Can you work these out from the model? Positions are in its coordinate system, mm. A direction names the side the tool comes from. Give positions to 0.01 mm unless a question says otherwise; leave off trailing zeros. Loops run counter-clockwise (first coordinate to the right, second up) from the corner with the lowest first, then second, coordinate; pieces in that order, holes last. Notation, with made-up numbers: (51.25, 39) - (107.25, 39) arc R18 cw to (107.25, 48) - close; hole circle Ø5 at (-9, 65.25). An arc over 180 degrees is marked (long way). Answer in a Markdown table with one row per item.
from build123d import *

# Parameters (mm, degrees)
SKETCH4_W                                       = 300
SKETCH4_H                                       = 100
BOSS_EXTRUDE2_DEPTH                             = 20
CSK_FOR_M2_FLAT_HEAD_MACHINE_SCREW1_D           = 2.4
CSK_FOR_M2_FLAT_HEAD_MACHINE_SCREW1_CSINK_D     = 4.4
CSK_FOR_M2_FLAT_HEAD_MACHINE_SCREW1_CSINK_ANGLE = 90
CBORE_FOR_M5_HEX_HEAD_BOLT1_D                   = 5.5
CBORE_FOR_M5_HEX_HEAD_BOLT1_CBORE_D             = 12.24
CBORE_FOR_M5_HEX_HEAD_BOLT1_CBORE_DEPTH         = 3.58


with BuildPart() as part:
    # Sketch4 → Boss-Extrude2 (new body)
    with BuildSketch(Plane(origin=(0, 0, 0), x_dir=(1, 0, 0), z_dir=(0, 1, 0))):
        Rectangle(SKETCH4_W, SKETCH4_H)
    extrude(amount=BOSS_EXTRUDE2_DEPTH)

    # CSK for M2 Flat Head Machine Screw1 (through all)
    with Locations(Plane(origin=(0, 20, 0), x_dir=(1, 0, 0), z_dir=(0, 1, 0))):
        with Locations((-120, 0), (-106, -0.273765591), (-112.818119913, 7.041508898), (-112.818119913, -6.958491102)):
            CounterSinkHole(CSK_FOR_M2_FLAT_HEAD_MACHINE_SCREW1_D / 2, CSK_FOR_M2_FLAT_HEAD_MACHINE_SCREW1_CSINK_D / 2, counter_sink_angle=CSK_FOR_M2_FLAT_HEAD_MACHINE_SCREW1_CSINK_ANGLE)

    # CBORE for M5 Hex Head Bolt1 (through all)
    with Locations(Plane(origin=(0, 0, -50), x_dir=(-1, 0, 0), z_dir=(0, 0, -1))):
        with Locations((0, 10), (-100, 10), (100, 10)):
            CounterBoreHole(CBORE_FOR_M5_HEX_HEAD_BOLT1_D / 2, CBORE_FOR_M5_HEX_HEAD_BOLT1_CBORE_D / 2, CBORE_FOR_M5_HEX_HEAD_BOLT1_CBORE_DEPTH)


solid = part.part
Q1. For pin 1 (4.5 mm diameter, centred on x = 0, y = 10, fed in from +Z); pin 2 (6 mm diameter, centred on x = -101.5, y = 7.5, fed in from -Z); pin 3 (4 mm diameter, centred on x = -120, z = 0, fed in from +Y); pin 4 (3 mm diameter, centred on x = -112.82, z = 6.96, fed in from +Y), each with a flat end and sliding along its axis, tell me the tip position at first contact or that it passes through.
Checked values:
| item | result |
|---|---|
| pin 1 | passes through |
| pin 2 | stops at z = -46.42 |
| pin 3 | stops at y = 19.8 |
| pin 4 | stops at y = 19.3 |
Q2. On a 3-axis mill with a long thin cutter (end or side, diameter ignored), from which of +Z, -Z, +X, -X, +Y, -Y can I reach the whole of each face in a straight line? I mean faces 4 (the face through (-105.837, 11.838, -48.235)), 5 (the face through (-2, 0, -1)). Say none if no direction works.
Checked values:
| item | result |
|---|---|
| face 4 | -Z |
| face 5 | +Z, -Z, +X, -X, -Y |
Q3. If I drill on line 1 (X direction, y = 12, z = -31); line 2 (X direction, y = 7.5, z = 5.5); line 3 (Z direction, x = -113.5, y = 2.25), over which ranges is the centre line in solid material (lowest first)? Write a range as [from, to].
Checked values:
| item | result |
|---|---|
| line 1 | x = [-150, -101.89], [-98.11, -1.89], [1.89, 98.11], [101.89, 150] |
| line 2 | x = [-150, -101.15], [-98.85, -1.15], [1.15, 98.85], [101.15, 150] |
| line 3 | z = [-50, -8.03], [-6.05, 5.97], [7.95, 50] |
Q4. Imagine slicing it at A-A, the plane x = 0. Write out the boundary of the cut face in (y, z).
Checked values:
| item | result |
|---|---|
| outline | (0, -50) - (3.88, -50) - (3.88, -46.42) - (7.25, -46.42) - (7.25, 50) - (0, 50) - close; (12.75, -46.42) - (16.12, -46.42) - (16.12, -50) - (20, -50) - (20, 50) - (12.75, 50) - close |
Q5. If we mould it in two halves opening along Y, with no side actions, what happens to faces 1 (the face through (-2, 3, -50)), 2 (the face through (-2, 20, -1)), 3 (the face through (-0.358, 12.727, 2.465))? For each: released by +Y, released by -Y, zero draft, split by the parting line, or undercut.
Checked values:
| item | result |
|---|---|
| face 1 | zero draft |
| face 2 | released by +Y |
| face 3 | undercut |
Q6. Imagine slicing it at B-B, the plane y = 10. Count the separate pieces of the cut face and the enclosed holes in it, and give its area (3 significant figures).
Checked values:
| item | result |
|---|---|
| separate pieces | 4 |
| enclosed holes | 4 |
| area | 28,300 mm² |
